Check sheet for the modelled part. Datum: model origin and axes. Units: mm. Face numbers are marked on the shaded views. Coordinates: 2 decimals unless noted, no trailing zeros. Order: outer loops, then holes, each group sorted by start corner. A loop starts at its lowest first (then second) coordinate and runs counter-clockwise, first axis right, second up. Notation, with made-up numbers: (-25, -23.5) -> (9, -23.5) arc R24 cw to (9, -7.5) -> close; hole circle Ø11 at (0.25, 76). An arc over 180 degrees is marked (long way). Put each result on its own line as item: value. Start each with the question number.
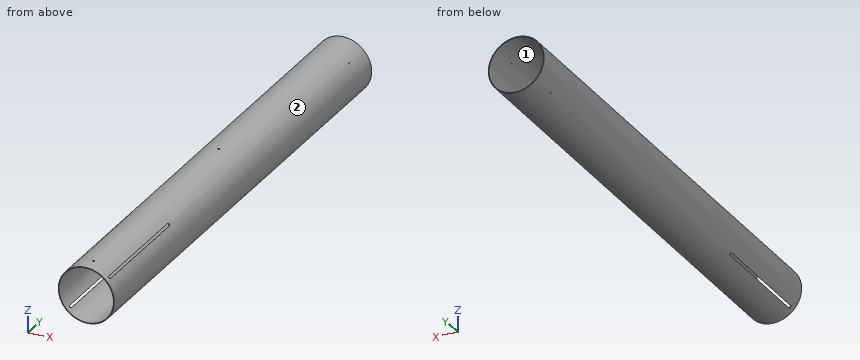
```python
from build123d import *

# Parameters (mm, degrees)
SKETCH1_R           = 50.8
SKETCH1_R_2         = 49.53
BOSS_EXTRUDE1_DEPTH = 889
CUT_EXTRUDE1_DEPTH  = 152.4
CIRPATTERN1_COUNT   = 4
SKETCH3_R           = 1.7653
CUT_EXTRUDE2_DEPTH  = 11.684
SKETCH4_R           = 1.0922
CUT_EXTRUDE3_DEPTH  = 25.4
CIRPATTERN2_COUNT   = 2


with BuildPart() as part:
    # Sketch1 → Boss-Extrude1 (new body)
    with BuildSketch(Plane(origin=(0, 0, 0), x_dir=(1, 0, 0), z_dir=(0, 1, 0))):
        with Locations(Location((0, 0, 0), (0, 0, 270))):
            Circle(SKETCH1_R)
        with Locations(Location((0, 0, 0), (0, 0, 270))):
            Circle(SKETCH1_R_2, mode=Mode.SUBTRACT)
    extrude(amount=BOSS_EXTRUDE1_DEPTH)

    # Sketch2 → Cut-Extrude1 (cut)
    with BuildSketch(Plane(origin=(10.001989034, 1243.355570529, -188.138382022), x_dir=(0, 1, 0), z_dir=(0.7071067811865634, 0, -0.7071067811865316))):
        with BuildLine():
            Line((-1230.655570529, 128.342701458), (-1027.455570529, 128.342701458))
            ThreePointArc((-1027.455570529, 128.342701458), (-1025.074320529, 125.961451458), (-1027.455570529, 123.580201458))
            Line((-1027.455570529, 123.580201458), (-1230.655570529, 123.580201458))
            ThreePointArc((-1230.655570529, 123.580201458), (-1233.036820529, 125.961451458), (-1230.655570529, 128.342701458))
        make_face()
    cut_extrude1 = extrude(amount=-CUT_EXTRUDE1_DEPTH, mode=Mode.SUBTRACT)

    # CirPattern1: Cut-Extrude1 ×4 about axis
    cirpattern1_axis = Axis((0, 0, 0), (0, 1, 0))
    for i in range(1, CIRPATTERN1_COUNT):
        add(cut_extrude1.rotate(cirpattern1_axis, i * 360 / CIRPATTERN1_COUNT), mode=Mode.SUBTRACT)

    # Sketch3 → Cut-Extrude2 (cut)
    with BuildSketch(Plane(origin=(271.091614788, 1243.355570529, 52.3875), x_dir=(-1, 0, 0), z_dir=(0, 0, 1))):
        with Locations(Location((271.091614788, 1217.955570529, 0), (0, 0, 180))):
            Circle(SKETCH3_R)
        with Locations(Location((271.091614788, 786.155570529, 0), (0, 0, 180))):
            Circle(SKETCH3_R)
    extrude(amount=-CUT_EXTRUDE2_DEPTH, mode=Mode.SUBTRACT)

    # Sketch4 → Cut-Extrude3 (cut)
    with BuildSketch(Plane(origin=(120.58027232, 708.404628356, -48.738223352), x_dir=(-0.7071067811865634, 2.660214291711019e-15, 0.7071067811865317), z_dir=(0.7071067811865317, -1.2152886494782433e-14, 0.7071067811865634))):
        with Locations(Location((119.72625647, -129.795371644, 0), (0, 0, 180))):
            Circle(SKETCH4_R)
    cut_extrude3 = extrude(amount=-CUT_EXTRUDE3_DEPTH, mode=Mode.SUBTRACT)

    # CirPattern2: Cut-Extrude3 ×2 about axis
    cirpattern2_axis = Axis((0, 889, 0), (0, -1, 0))
    for i in range(1, CIRPATTERN2_COUNT):
        add(cut_extrude3.rotate(cirpattern2_axis, i * 360 / CIRPATTERN2_COUNT), mode=Mode.SUBTRACT)


solid = part.part
```
1) Sectioned sample at C-C (y = 512.5). Record the boundary of the cut face in (x, z), plus the area to 3 significant figures.
2) Mould release check, pull along X, two halves, no side actions. Record for the marked faces 1 and 2: +X half, -X half, draft (parallel to the pull), parting line (faces both ways), or undercut.
3) Sectioned sample at B-B (z = 0). Record the boundary of the cut face in (x, y), plus the area to 3 significant figures.
4) Gauge pin test, flat ends, axial feed: pin 1 (1.5 mm diameter, centred on y = 336.5, z = -33, fed in from +X); pin 2 (1.5 mm diameter, centred on x = 26, y = 586, fed in from +Z); pin 3 (6 mm diameter, centred on y = 272, z = -28, fed in from -X). Record the tip position at first contact, or that the pin passes through.
5) Scan lines: line 1 along Y through (x, z) = (0, 49.85); line 2 along X through (y, z) = (667.5, 0); line 3 along Z through (x, y) = (-1, 307.5). Record each from-to range of solid material in increasing order. Write a range as [from, to].
6) Sectioned sample at A-A (y = 151). Record the boundary of the cut face in (x, z).
Entries:
1. outline: circle Ø101.6 at (0, 0); hole circle Ø99.06 at (0, 0)
1. area: 400 mm2
2. face 1: undercut
2. face 2: parting line
3. outline: (-50.8, 0) -> (-49.53, 0) -> (-49.53, 889) -> (-50.8, 889) -> close; (49.53, 0) -> (50.8, 0) -> (50.8, 889) -> (49.53, 889) -> close
3. area: 2,260 mm2
4. pin 1: stops at x = 39.25
4. pin 2: stops at z = 44.08
4. pin 3: stops at x = -44.22
5. line 1: y = [0, 23.63], [27.17, 455.43], [458.97, 889]
5. line 2: x = [-50.8, -49.53], [49.53, 50.8]
5. line 3: z = [-50.79, -49.52], [49.52, 50.79]
6. outline: (-37.57, -34.2) -> (-36.67, -33.3) arc R49.53 cw to (-36.67, 33.3) -> (-37.57, 34.2) arc R50.8 ccw to start; (-34.2, -37.57) arc R50.8 ccw to (34.2, -37.57) -> (33.3, -36.67) arc R49.53 cw to (-33.3, -36.67) -> close; (-34.2, 37.57) -> (-33.3, 36.67) arc R49.53 cw to (33.3, 36.67) -> (34.2, 37.57) arc R50.8 ccw to start; (36.67, -33.3) -> (37.57, -34.2) arc R50.8 ccw to (37.57, 34.2) -> (36.67, 33.3) arc R49.53 cw to start
